from build123d import *

# Parameters (mm, degrees)
F0_W     = 61
F0_H     = 75
F1_DEPTH = 20.5
F2_R     = 2
F3_T     = -2.5
F4_W     = 40
F4_H     = 14
F5_DEPTH = 25


with BuildPart() as f1:
    # F0 (on Front) → F1 (new body)
    with BuildSketch(Plane.XZ):
        with Locations((30.5, 37.5)):
            Rectangle(F0_W, F0_H)
    extrude(amount=F1_DEPTH)

    # F2
    f2_edges = [f1.edges().sort_by_distance(p)[0] for p in [
        (0, -10.25, 75),
        (61, -10.25, 75),
        (61, -10.25, 0),
        (0, -10.25, 0),
    ]]
    fillet(f2_edges, radius=F2_R)

    # F3
    f3_openings = [f1.faces().sort_by_distance(p)[0] for p in [
        (30.5, -20.5, 37.5),
    ]]
    offset(amount=F3_T, openings=f3_openings)

    # F4 (on face) → F5 (cut)
    with BuildSketch(Plane.XY.offset(2.5)):
        with Locations((32.5, -13.5)):
            Rectangle(F4_W, F4_H)
    extrude(amount=-F5_DEPTH, mode=Mode.SUBTRACT)


solid = f1.part
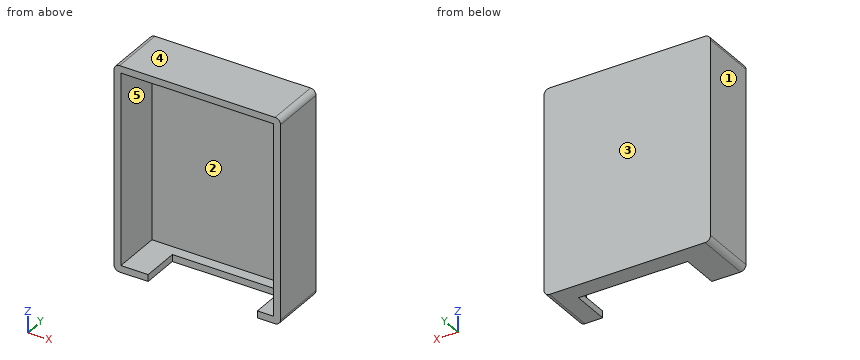
Read the model definition and answer for the solid it produces. Units are mm, in the model's axes. Face numbers are marked on the shaded views. A direction names the side the tool comes from. Round coordinates to 2 decimals unless told otherwise and drop trailing zeros. Order: outer loops, then holes, each group sorted by start corner. A loop starts at its lowest first (then second) coordinate and runs counter-clockwise, first axis right, second up.
1) For the marked faces 1 and 2, determine the directions among +Z, -Z, +X, -X, +Y, -Y from which every point of the face is accessible in a straight line to the end or side of a thin tool.
2) Straight lines are drawn through the part: L1, parallel to X at y = -17.75, z = 21.5; L2, parallel to Z at x = 24.5, y = -5.5; L3, parallel to Y at x = 36, z = 69. For each, find the intervals that lie inside material, in ascending order.
3) The part is cut by section B-B on x = 36. Write down the section's boundary in (y, z).
4) The part is cut by section D-D on y = -5.25. Write down the section's boundary in (x, z), plus the area to 3 significant figures.
5) The mould has two halves that part along Z. Classify the marked faces 3, 4 and 5: released by +Z, released by -Z, zero draft, split by the parting line, or undercut.
6) The part is cut by section C-C on y = -10.5. Write down the section's boundary in (x, z), plus the area to 3 significant figures.
7) The part is cut by section A-A on z = 6. Write down the section's boundary in (x, y).
8) Flat-ended cylindrical pins translate along their axes: pin 1 (5.5 mm diameter, centred on x = 33, y = -13, fed in from -Z); pin 2 (2 mm diameter, centred on x = 36.5, z = 1.5, fed in from -Y); pin 3 (3 mm diameter, centred on x = 53, z = 51.5, fed in from -Y). Find the tip coordinate at first contact, or state that the pin passes through.
Resolved:
1. face 1: +Z, -Z, -X, +Y, -Y
1. face 2: -Y
2. L1: x = 0 to 2.5, 58.5 to 61
2. L2: z = 0 to 2.5, 72.5 to 75
2. L3: y = -2.5 to 0
3. outline: (-20.5, 72.5) - (-2.5, 72.5) - (-2.5, 2.5) - (-6.5, 2.5) - (-6.5, 0) - (0, 0) - (0, 75) - (-20.5, 75) - close
4. outline: (0, 2) arc R2 ccw to (2, 0) - (59, 0) arc R2 ccw to (61, 2) - (61, 73) arc R2 ccw to (59, 75) - (2, 75) arc R2 ccw to (0, 73) - close; hole (2.5, 2.5) - (58.5, 2.5) - (58.5, 72.5) - (2.5, 72.5) - close
4. area: 652 mm2
5. face 3: zero draft
5. face 4: released by +Z
5. face 5: undercut
6. outline: (0, 2) arc R2 ccw to (2, 0) - (12.5, 0) - (12.5, 2.5) - (2.5, 2.5) - (2.5, 72.5) - (58.5, 72.5) - (58.5, 2.5) - (52.5, 2.5) - (52.5, 0) - (59, 0) arc R2 ccw to (61, 2) - (61, 73) arc R2 ccw to (59, 75) - (2, 75) arc R2 ccw to (0, 73) - close
6. area: 552 mm2
7. outline: (0, -20.5) - (2.5, -20.5) - (2.5, -2.5) - (58.5, -2.5) - (58.5, -20.5) - (61, -20.5) - (61, 0) - (0, 0) - close
8. pin 1: stops at z = 72.5
8. pin 2: stops at y = -6.5
8. pin 3: stops at y = -2.5
